Check sheet for the modelled part. Datum: model origin and axes. Units: mm. A direction names the side the tool comes from. Give positions to 0.01 mm unless a question says otherwise; leave off trailing zeros. Write each loop counter-clockwise with the first axis right and the second up, starting at its lowest first coordinate (ties: lowest second). Pieces come first, ordered by that corner, then holes. Notation, with made-up numbers: (17, 25.5) -> (36, 25.5) arc R7 ccw to (36, 38.5) -> close; hole circle Ø9 at (38.5, -21). An arc over 180 degrees is marked (long way). Return JSON: item names as keys, results as strings.
from build123d import *

# Parameters (mm, degrees)
F0_W      = 200
F0_H      = 400
F1_DEPTH  = 30
F3_DEPTH  = 30
F4_W      = 50
F4_H      = 62
F5_DEPTH  = 10
F6_R      = 6
F7_DEPTH  = 8
F9_DEPTH  = 30
F10_W     = 200
F10_H     = 121.5
F11_DEPTH = 30


with BuildPart() as f1:
    # F0 (on Front) → F1 (new body)
    with BuildSketch(Plane.XZ):
        with Locations((100, 200)):
            Rectangle(F0_W, F0_H)
    extrude(amount=F1_DEPTH)

    # F2 (on face) → F3 (cut)
    with BuildSketch(Plane.XZ.offset(30)):
        with BuildLine():
            ThreePointArc((23, 185), (17.8786796564, 187.1213203436), (20, 182))
            Line((20, 182), (20, 185))
            Line((20, 185), (23, 185))
        make_face()
        with BuildLine():
            Line((20, 185), (20, 182))
            ThreePointArc((20, 182), (22.1213203436, 182.8786796564), (23, 185))
            Line((23, 185), (20, 185))
        make_face()
        with BuildLine():
            ThreePointArc((20, 153), (17, 150), (20, 147))
            Line((20, 147), (20, 150))
            Line((20, 150), (20, 153))
        make_face()
        with BuildLine():
            Line((20, 153), (20, 150))
            Line((20, 150), (23, 150))
            ThreePointArc((23, 150), (22.1213203436, 152.1213203436), (20, 153))
        make_face()
        with BuildLine():
            Line((20, 150), (20, 147))
            ThreePointArc((20, 147), (22.1213203436, 147.8786796564), (23, 150))
            Line((23, 150), (20, 150))
        make_face()
        with BuildLine():
            Line((55, 150), (52, 150))
            ThreePointArc((52, 150), (52.8786796564, 147.8786796564), (55, 147))
            Line((55, 147), (55, 150))
        make_face()
        with BuildLine():
            ThreePointArc((55, 153), (52.8786796564, 152.1213203436), (52, 150))
            Line((52, 150), (55, 150))
            Line((55, 150), (55, 153))
        make_face()
        with BuildLine():
            Line((55, 150), (55, 147))
            ThreePointArc((55, 147), (57.1213203436, 147.8786796564), (58, 150))
            ThreePointArc((58, 150), (57.1213203436, 152.1213203436), (55, 153))
            Line((55, 153), (55, 150))
        make_face()
        with BuildLine():
            Line((55, 185), (52, 185))
            ThreePointArc((52, 185), (52.8786796564, 182.8786796564), (55, 182))
            Line((55, 182), (55, 185))
        make_face()
        with BuildLine():
            ThreePointArc((58, 185), (55, 188), (52, 185))
            Line((52, 185), (55, 185))
            Line((55, 185), (55, 182))
            ThreePointArc((55, 182), (57.1213203436, 182.8786796564), (58, 185))
        make_face()
        with BuildLine():
            ThreePointArc((148, 185), (142.8786796564, 187.1213203436), (145, 182))
            Line((145, 182), (145, 185))
            Line((145, 185), (148, 185))
        make_face()
        with BuildLine():
            Line((145, 185), (145, 182))
            ThreePointArc((145, 182), (147.1213203436, 182.8786796564), (148, 185))
            Line((148, 185), (145, 185))
        make_face()
        with BuildLine():
            ThreePointArc((177, 185), (177.8786796564, 182.8786796564), (180, 182))
            Line((180, 182), (180, 185))
            Line((180, 185), (177, 185))
        make_face()
        with BuildLine():
            Line((180, 185), (180, 182))
            ThreePointArc((180, 182), (182.1213203436, 182.8786796564), (183, 185))
            ThreePointArc((183, 185), (180, 188), (177, 185))
            Line((177, 185), (180, 185))
        make_face()
        with BuildLine():
            ThreePointArc((177, 150), (177.8786796564, 147.8786796564), (180, 147))
            Line((180, 147), (180, 150))
            Line((180, 150), (177, 150))
        make_face()
        with BuildLine():
            Line((177, 150), (180, 150))
            Line((180, 150), (180, 153))
            ThreePointArc((180, 153), (177.8786796564, 152.1213203436), (177, 150))
        make_face()
        with BuildLine():
            Line((180, 150), (180, 147))
            ThreePointArc((180, 147), (182.1213203436, 147.8786796564), (183, 150))
            ThreePointArc((183, 150), (182.1213203436, 152.1213203436), (180, 153))
            Line((180, 153), (180, 150))
        make_face()
        with BuildLine():
            Line((145, 150), (145, 147))
            ThreePointArc((145, 147), (147.1213203436, 147.8786796564), (148, 150))
            Line((148, 150), (145, 150))
        make_face()
        with BuildLine():
            Line((145, 153), (145, 150))
            Line((145, 150), (148, 150))
            ThreePointArc((148, 150), (147.1213203436, 152.1213203436), (145, 153))
        make_face()
        with BuildLine():
            ThreePointArc((145, 153), (142, 150), (145, 147))
            Line((145, 147), (145, 150))
            Line((145, 150), (145, 153))
        make_face()
        with BuildLine():
            Line((180, 45), (180, 42))
            ThreePointArc((180, 42), (182.1213203436, 42.8786796564), (183, 45))
            ThreePointArc((183, 45), (182.1213203436, 47.1213203436), (180, 48))
            Line((180, 48), (180, 45))
        make_face()
        with BuildLine():
            ThreePointArc((177, 45), (177.8786796564, 42.8786796564), (180, 42))
            Line((180, 42), (180, 45))
            Line((180, 45), (177, 45))
        make_face()
        with BuildLine():
            Line((177, 45), (180, 45))
            Line((180, 45), (180, 48))
            ThreePointArc((180, 48), (177.8786796564, 47.1213203436), (177, 45))
        make_face()
        with BuildLine():
            Line((145, 45), (145, 42))
            ThreePointArc((145, 42), (147.1213203436, 42.8786796564), (148, 45))
            Line((148, 45), (145, 45))
        make_face()
        with BuildLine():
            Line((145, 45), (148, 45))
            ThreePointArc((148, 45), (147.1213203436, 47.1213203436), (145, 48))
            Line((145, 48), (145, 45))
        make_face()
        with BuildLine():
            ThreePointArc((145, 48), (142, 45), (145, 42))
            Line((145, 42), (145, 45))
            Line((145, 45), (145, 48))
        make_face()
        with BuildLine():
            ThreePointArc((145, 13), (142.8786796564, 7.8786796564), (148, 10))
            Line((148, 10), (145, 10))
            Line((145, 10), (145, 13))
        make_face()
        with BuildLine():
            Line((145, 10), (148, 10))
            ThreePointArc((148, 10), (147.1213203436, 12.1213203436), (145, 13))
            Line((145, 13), (145, 10))
        make_face()
        with BuildLine():
            ThreePointArc((177, 10), (177.8786796564, 7.8786796564), (180, 7))
            Line((180, 7), (180, 10))
            Line((180, 10), (177, 10))
        make_face()
        with BuildLine():
            Line((180, 13), (180, 10))
            Line((180, 10), (183, 10))
            ThreePointArc((183, 10), (182.1213203436, 12.1213203436), (180, 13))
        make_face()
        with BuildLine():
            Line((177, 10), (180, 10))
            Line((180, 10), (180, 13))
            ThreePointArc((180, 13), (177.8786796564, 12.1213203436), (177, 10))
        make_face()
        with BuildLine():
            Line((180, 10), (180, 7))
            ThreePointArc((180, 7), (182.1213203436, 7.8786796564), (183, 10))
            Line((183, 10), (180, 10))
        make_face()
        with BuildLine():
            Line((17, 10), (20, 10))
            Line((20, 10), (20, 13))
            ThreePointArc((20, 13), (17.8786796564, 12.1213203436), (17, 10))
        make_face()
        with BuildLine():
            Line((20, 7), (20, 10))
            Line((20, 10), (17, 10))
            ThreePointArc((17, 10), (17.8786796564, 7.8786796564), (20, 7))
        make_face()
        with BuildLine():
            Line((23, 10), (20, 10))
            Line((20, 10), (20, 7))
            ThreePointArc((20, 7), (22.1213203436, 7.8786796564), (23, 10))
        make_face()
        with BuildLine():
            Line((20, 13), (20, 10))
            Line((20, 10), (23, 10))
            ThreePointArc((23, 10), (22.1213203436, 12.1213203436), (20, 13))
        make_face()
        with BuildLine():
            Line((55, 10), (52, 10))
            ThreePointArc((52, 10), (55, 7), (58, 10))
            ThreePointArc((58, 10), (57.1213203436, 12.1213203436), (55, 13))
            Line((55, 13), (55, 10))
        make_face()
        with BuildLine():
            ThreePointArc((55, 13), (52.8786796564, 12.1213203436), (52, 10))
            Line((52, 10), (55, 10))
            Line((55, 10), (55, 13))
        make_face()
        with BuildLine():
            Line((55, 45), (55, 42))
            ThreePointArc((55, 42), (57.1213203436, 42.8786796564), (58, 45))
            ThreePointArc((58, 45), (57.1213203436, 47.1213203436), (55, 48))
            Line((55, 48), (55, 45))
        make_face()
        with BuildLine():
            ThreePointArc((52, 45), (52.8786796564, 42.8786796564), (55, 42))
            Line((55, 42), (55, 45))
            Line((55, 45), (52, 45))
        make_face()
        with BuildLine():
            ThreePointArc((55, 48), (52.8786796564, 47.1213203436), (52, 45))
            Line((52, 45), (55, 45))
            Line((55, 45), (55, 48))
        make_face()
        with BuildLine():
            Line((20, 45), (20, 42))
            ThreePointArc((20, 42), (22.1213203436, 42.8786796564), (23, 45))
            Line((23, 45), (20, 45))
        make_face()
        with BuildLine():
            ThreePointArc((20, 48), (17, 45), (20, 42))
            Line((20, 42), (20, 45))
            Line((20, 45), (20, 48))
        make_face()
        with BuildLine():
            Line((20, 48), (20, 45))
            Line((20, 45), (23, 45))
            ThreePointArc((23, 45), (22.1213203436, 47.1213203436), (20, 48))
        make_face()
    extrude(amount=-F3_DEPTH, mode=Mode.SUBTRACT)

    # F4 (on face) → F5 (cut)
    with BuildSketch(Plane.XZ.offset(30)):
        with Locations((100, 97.5)):
            Rectangle(F4_W, F4_H)
    extrude(amount=-F5_DEPTH, mode=Mode.SUBTRACT)

    # F6 (on face) → F7 (cut)
    with BuildSketch(Plane(origin=(0, 0, 0), x_dir=(-1, 0, 0), z_dir=(0, 1, 0))):
        with Locations((-180, 185)):
            Circle(F6_R)
        with Locations((-180, 150)):
            Circle(F6_R)
        with Locations((-145, 185)):
            Circle(F6_R)
        with Locations((-145, 150)):
            Circle(F6_R)
        with Locations((-180, 45)):
            Circle(F6_R)
        with Locations((-180, 10)):
            Circle(F6_R)
        with Locations((-145, 45)):
            Circle(F6_R)
        with Locations((-145, 10)):
            Circle(F6_R)
        with Locations((-55, 185)):
            Circle(F6_R)
        with Locations((-55, 150)):
            Circle(F6_R)
        with Locations((-20, 185)):
            Circle(F6_R)
        with Locations((-20, 150)):
            Circle(F6_R)
        with Locations((-55, 45)):
            Circle(F6_R)
        with Locations((-55, 10)):
            Circle(F6_R)
        with Locations((-20, 45)):
            Circle(F6_R)
        with Locations((-20, 10)):
            Circle(F6_R)
    extrude(amount=-F7_DEPTH, mode=Mode.SUBTRACT)

    # F8 (on face) → F9 (cut)
    with BuildSketch(Plane.XZ.offset(20)):
        with BuildLine():
            Line((93, 121.5), (93, 118.5))
            ThreePointArc((93, 118.5), (95.1213203436, 119.3786796564), (96, 121.5))
            Line((96, 121.5), (93, 121.5))
        make_face()
        with BuildLine():
            ThreePointArc((96, 121.5), (90.8786796564, 123.6213203436), (93, 118.5))
            Line((93, 118.5), (93, 121.5))
            Line((93, 121.5), (96, 121.5))
        make_face()
        with BuildLine():
            ThreePointArc((114, 121.5), (114.8786796564, 119.3786796564), (117, 118.5))
            Line((117, 118.5), (117, 121.5))
            Line((117, 121.5), (114, 121.5))
        make_face()
        with BuildLine():
            Line((117, 121.5), (117, 118.5))
            ThreePointArc((117, 118.5), (119.1213203436, 119.3786796564), (120, 121.5))
            ThreePointArc((120, 121.5), (117, 124.5), (114, 121.5))
            Line((114, 121.5), (117, 121.5))
        make_face()
        with BuildLine():
            Line((96, 73.5), (93, 73.5))
            Line((93, 73.5), (93, 76.5))
            ThreePointArc((93, 76.5), (90.8786796564, 71.3786796564), (96, 73.5))
        make_face()
        with BuildLine():
            Line((93, 76.5), (93, 73.5))
            Line((93, 73.5), (96, 73.5))
            ThreePointArc((96, 73.5), (95.1213203436, 75.6213203436), (93, 76.5))
        make_face()
        with BuildLine():
            ThreePointArc((117, 76.5), (114.8786796564, 75.6213203436), (114, 73.5))
            Line((114, 73.5), (117, 73.5))
            Line((117, 73.5), (117, 76.5))
        make_face()
        with BuildLine():
            Line((117, 73.5), (114, 73.5))
            ThreePointArc((114, 73.5), (117, 70.5), (120, 73.5))
            ThreePointArc((120, 73.5), (119.1213203436, 75.6213203436), (117, 76.5))
            Line((117, 76.5), (117, 73.5))
        make_face()
    extrude(amount=-F9_DEPTH, mode=Mode.SUBTRACT)

    # F10 (on face) → F11 (cut)
    with BuildSketch(Plane(origin=(0, 0, 0), x_dir=(-1, 0, 0), z_dir=(0, 1, 0))):
        with Locations((-100, 339.25)):
            Rectangle(F10_W, F10_H)
    extrude(amount=-F11_DEPTH, mode=Mode.SUBTRACT)


solid = f1.part
(1) Cross-section at B-B on z = 107. Enter the section's corners in (x, y).
Reply:
{"outline": "(0, -30) -> (75, -30) -> (75, -20) -> (125, -20) -> (125, -30) -> (200, -30) -> (200, 0) -> (0, 0) -> close"}
(2) Cross-section at A-A on y = -4.75. State how many separate pieces and enclosed holes the cut face has, then the cut area to 3 significant figures.
Reply:
{"separate pieces": "1", "enclosed holes": "20", "area": "53,800 mm^2"}
(3) Release check for a two-part mould opening along Z. For faces 3 (the flat face through (148, -8, 44)), 4 (the flat face through (19, -8, 188)), 5 (the flat face through (99, -30, 141)) record: pulls with the +Z half, pulls with the -Z half, needs draft (parallel to the pull), parting line crosses it, or undercut.
Reply:
{"face 3": "undercut", "face 4": "undercut", "face 5": "needs draft"}
(4) Cross-section at C-C on x = 83. Enter the section's corners in (y, z), then the cut area to 4 significant figures.
Reply:
{"outline": "(-30, 0) -> (0, 0) -> (0, 278.5) -> (-30, 278.5) -> (-30, 128.5) -> (-20, 128.5) -> (-20, 66.5) -> (-30, 66.5) -> close", "area": "7,735 mm^2"}
(5) Thickness scan on L1, parallel to Z at x = 145, y = -1.75; L2, parallel to X at y = -12.75, z = 185; L3, parallel to X at y = -10, z = 121.5. Record the ranges inside material, lowest first.
Reply:
{"L1": "0 to 4, 16 to 39, 51 to 144, 156 to 179, 191 to 278.5", "L2": "0 to 17, 23 to 52, 58 to 142, 148 to 177, 183 to 200", "L3": "0 to 90, 96 to 114, 120 to 200"}
(6) Set-up check for faces 1 (the cylindrical face through (21.301, -3.944, 179.143)), 2 (the flat face through (100, -20, 98)): record each of +Z, -Z, +X, -X, +Y, -Y from which the full face is reachable in a straight line by a thin tool's end or side.
Reply:
{"face 1": "+Y", "face 2": "-Y"}
(7) Depth check by flat-ended pin: pin 1 Ø15.5 at (x, z) = (20, 45) entering from -Y; pin 2 Ø8 at (x, z) = (93, 73.5) entering from -Y; pin 3 Ø6 at (x, z) = (180.5, 11.5) entering from +Y. Enter the tip coordinate at first touch or a pass-through.
Reply:
{"pin 1": "y = -30", "pin 2": "y = -20", "pin 3": "y = -8"}
